from build123d import *


with BuildPart() as f1:
    # F0 (on Top) → F1 (revolve)
    with BuildSketch(Plane.XY):
        with BuildLine():
            Line((0, 6.00075), (0, 0))
            Line((0, 0), (76.2, 0))
            Line((76.2, 0), (76.2, 6.00075))
            Line((76.2, 6.00075), (56.769, 6.00075))
            ThreePointArc((56.769, 6.00075), (55.1815, 4.41325), (53.594, 6.00075))
            Line((53.594, 6.00075), (21.844, 6.00075))
            ThreePointArc((21.844, 6.00075), (20.2565, 4.41325), (18.669, 6.00075))
            Line((18.669, 6.00075), (0, 6.00075))
        make_face()
    revolve(axis=Axis((38.1, 0, 0), (1, 0, 0)))


solid = f1.part
Check sheet for the modelled part. Datum: model origin and axes. Units: mm. Round coordinates to 2 decimals unless told otherwise and drop trailing zeros. Order: outer loops, then holes, each group sorted by start corner. A loop starts at its lowest first (then second) coordinate and runs counter-clockwise, first axis right, second up.
(1) Cross-section at C-C, the plane x = 69. Enter the section's corners in (y, z).
(2) Cross-section at A-A, the plane z = 0. Enter the section's corners in (x, y) (1 decimal).
(3) Cross-section at D-D, the plane z = 4.75. State how many separate pieces and enclosed holes the cut face has, and give its area (3 significant figures).
(4) Scan lines: probe 1 along X at (y, z) = (4.5, -2.5); probe 2 along X at (y, z) = (3.5, 4); probe 3 along Y at (x, z) = (73, 0.5). Record each from-to range of solid material in increasing order.
Check sheet entries:
1. outline: circle Ø12 at (0, 0)
2. outline: (0, -6) - (18.7, -6) arc R1.6 cw to (21.8, -6) - (53.6, -6) arc R1.6 cw to (56.8, -6) - (76.2, -6) - (76.2, 6) - (56.8, 6) arc R1.6 cw to (53.6, 6) - (21.8, 6) arc R1.6 cw to (18.7, 6) - (0, 6) - close
3. separate pieces: 3
3. enclosed holes: 0
3. area: 521 mm2
4. probe 1: x = 0 to 18.92, 21.6 to 53.84, 56.52 to 76.2
4. probe 2: x = 0 to 18.82, 21.69 to 53.75, 56.61 to 76.2
4. probe 3: y = -5.98 to 5.98
